Design review of the part shown in the three views and the two pictorial views. Dimensions are in mm from the part's minimum x, y and z. A direction names the side the tool comes from. Give positions to 0.01 mm unless a question says otherwise; leave off trailing zeros. Loops run counter-clockwise (first coordinate to the right, second up) from the corner with the lowest first, then second, coordinate; pieces in that order, holes last. Notation, with made-up numbers: (19.5, 34.25) - (31.5, 34.25) arc R26 cw to (31.5, 58.25) - close; hole circle Ø3 at (28, 19.25). An arc over 180 degrees is marked (long way). Answer as a JSON object with one key per item and string values.
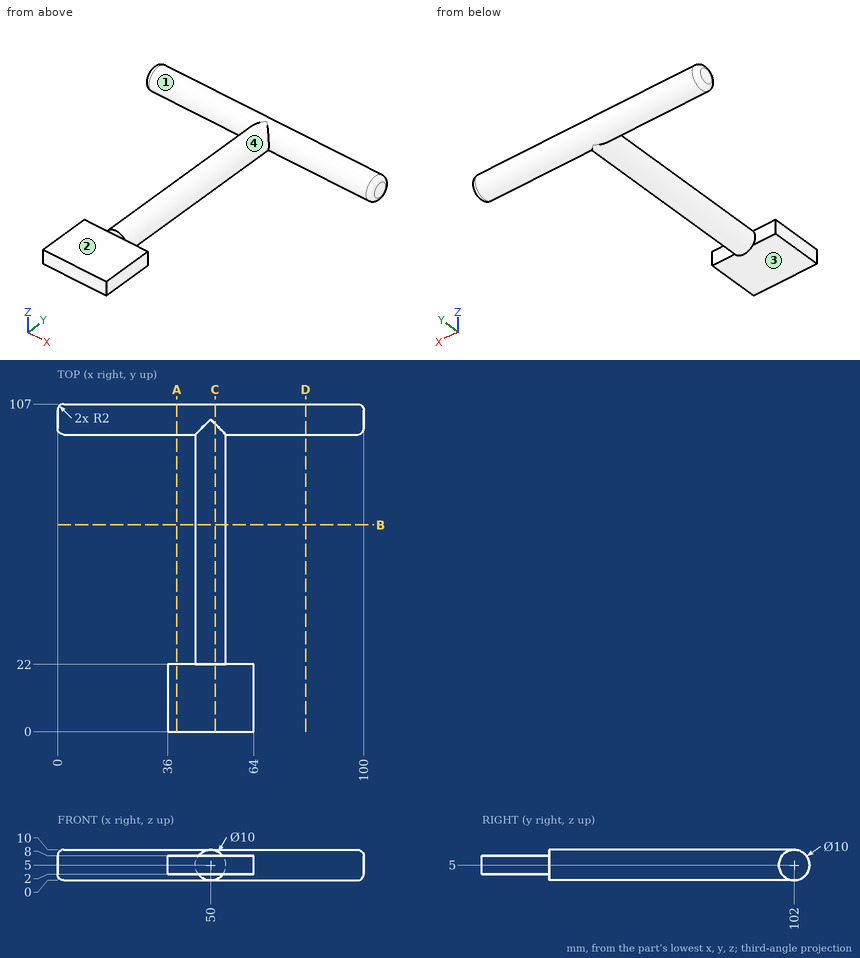
Q1. Consider section C-C, the plane x = 51.5. State the section outline as (y, z) points.
Results:
{"outline": "(0, 2) - (22, 2) - (22, 0.23) - (100.5, 0.23) arc R5 ccw (long way) to (100.5, 9.77) - (22, 9.77) - (22, 8) - (0, 8) - close"}
Q2. The part is to be moulded in two halves that separate along Y. For the marked faces 3 and 4, say which applies: +Y half, -Y half, draft (parallel to the pull), parting line (faces both ways), or undercut.
Results:
{"face 3": "draft", "face 4": "undercut"}
Q3. Clearance check with flat-ended pins moving along their axes: pin 1 Ø3 at (y, z) = (10.5, 6) entering from -X; pin 2 Ø3 at (y, z) = (13, 4.5) entering from +X; pin 3 Ø4 at (y, z) = (79, 8.5) entering from +X. State where each tip first meets the part, or that it passes through.
Results:
{"pin 1": "stops at x = 36", "pin 2": "stops at x = 64", "pin 3": "stops at x = 54.77"}
Q4. For the marked faces 1 and 2, list the 3-axis set-ups (+Z, -Z, +X, -X, +Y, -Y) from which the entire face can be reached by the end or side of a thin tool; tool diameter is ignored.
Results:
{"face 1": "none", "face 2": "+Z, +X, -X, -Y"}
Q5. Consider section D-D, the plane x = 81. State the section outline as (y, z) points.
Results:
{"outline": "circle Ø10 at (102, 5)"}
Q6. Consider section B-B, the plane y = 67.5. State the section outline as (x, z) points.
Results:
{"outline": "circle Ø10 at (50, 5)"}
Q7. To check wall thickness, follow probe 1 along Y at (x, z) = (19.5, 9); probe 2 along X at (y, z) = (12, 6); probe 3 along X at (y, z) = (94, 2). State the ranges of each line that lie inside material, in increasing order. Write a range as [from, to].
Results:
{"probe 1": "y = [99, 105]", "probe 2": "x = [36, 64]", "probe 3": "x = [46, 54]"}
Q8. Consider section A-A, the plane x = 39. State the section outline as (y, z) points, plus the area to 3 significant figures.
Results:
{"outline": "(0, 2) - (22, 2) - (22, 8) - (0, 8) - close; circle Ø10 at (102, 5)", "area": "211 mm^2"}
